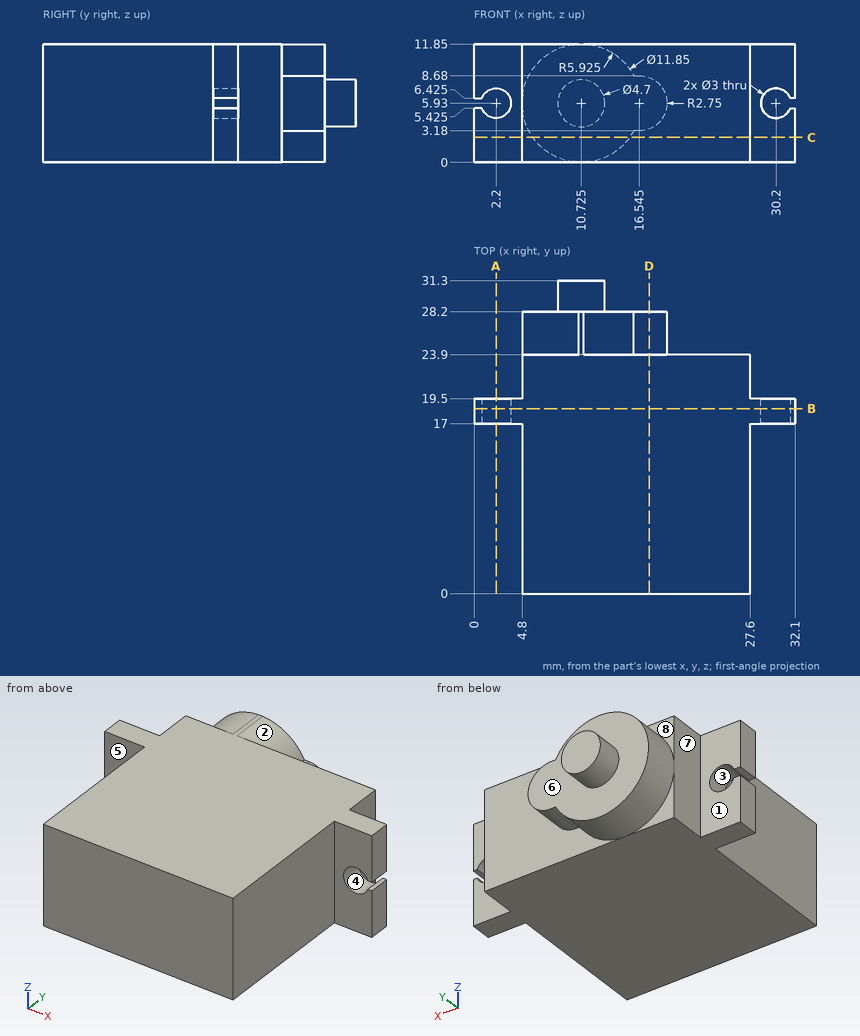
Verification items for this drawing (mm, ordinates from the low corner). A direction names the side the tool comes from. Round coordinates to 2 decimals unless told otherwise and drop trailing zeros. Order: outer loops, then holes, each group sorted by start corner. A loop starts at its lowest first (then second) coordinate and runs counter-clockwise, first axis right, second up. Notation, with made-up numbers: (-5.75, -5) - (44.25, -5) arc R6 cw to (44.25, 6) - close; hole circle Ø1 at (8, 18.5). An arc over 180 degrees is marked (long way). Use CSV: the item, a comma, the result in double quotes. Start each with the question number.
1) Mould release check, pull along Z, two halves, no side actions. Record for the marked faces 1, 2, 3 and 4: +Z half, -Z half, draft (parallel to the pull), parting line (faces both ways), or undercut.
2) Section check B-B, the plane y = 18.5. Record the cut outline in (x, z) (3 decimals), plus the area to 3 significant figures.
3) Thickness scan on L1, parallel to Z at x = 2.2, y = 17.65; L2, parallel to Y at x = 2, z = 1.25; L3, parallel to X at y = 7.5, z = 11. Record the ranges inside material, lowest first.
4) Section check A-A, the plane x = 2.2. Record the cut outline in (y, z), plus the area to 3 significant figures.
5) Section check C-C, the plane z = 2.5. Record the cut outline in (x, y).
6) Go/stop test with flat-tipped pins: P1, Ø6, axis at x = 5, z = 8.5, coming from the +Y side; P2, Ø1.4, axis at x = 29, z = 8, coming from the +Y side; P3, Ø0.6, axis at x = 16.5, y = 27, coming from the +Z side. Record where each tip stops, or that it passes through.
7) Access from +Z, -Z, +X, -X, +Y, -Y to the whole of each face (thin tool, end or side, straight path). Record for the marked faces 5, 6, 7 and 8.
8) Section check D-D, the plane x = 17.5. Record the cut outline in (y, z), plus the area to 3 significant figures.
Answers:
1,face 1,"draft"
1,face 2,"+Z half"
1,face 3,"undercut"
1,face 4,"undercut"
2,outline,"(0, 0) - (32.1, 0) - (32.1, 5.425) - (31.612, 5.425) arc R1.5 cw (long way) to (31.616, 6.425) - (32.1, 6.425) - (32.1, 11.85) - (0, 11.85) - (0, 6.425) - (0.784, 6.425) arc R1.5 cw (long way) to (0.788, 5.425) - (0, 5.425) - close"
2,area,"365 mm²"
3,L1,"z = 0 to 4.43, 7.43 to 11.85"
3,L2,"y = 17 to 19.5"
3,L3,"x = 4.8 to 27.6"
4,outline,"(17, 0) - (19.5, 0) - (19.5, 4.43) - (17, 4.43) - close; (17, 7.43) - (19.5, 7.43) - (19.5, 11.85) - (17, 11.85) - close"
4,area,"22.1 mm²"
5,outline,"(0, 17) - (4.8, 17) - (4.8, 0) - (27.6, 0) - (27.6, 17) - (32.1, 17) - (32.1, 19.5) - (27.6, 19.5) - (27.6, 23.9) - (15.56, 23.9) - (15.56, 28.2) - (5.89, 28.2) - (5.89, 23.9) - (4.8, 23.9) - (4.8, 19.5) - (0, 19.5) - close"
6,P1,"stops at y = 28.2"
6,P2,"stops at y = 19.5"
6,P3,"stops at z = 8.68"
7,face 5,"+Z, -Z, -X, -Y"
7,face 6,"+Y"
7,face 7,"+Z, -Z, -X, +Y"
7,face 8,"+Z, -X, +Y"
8,outline,"(0, 0) - (23.9, 0) - (23.9, 3.35) - (28.2, 3.35) - (28.2, 8.51) - (23.9, 8.51) - (23.9, 11.85) - (0, 11.85) - close"
8,area,"305 mm²"
